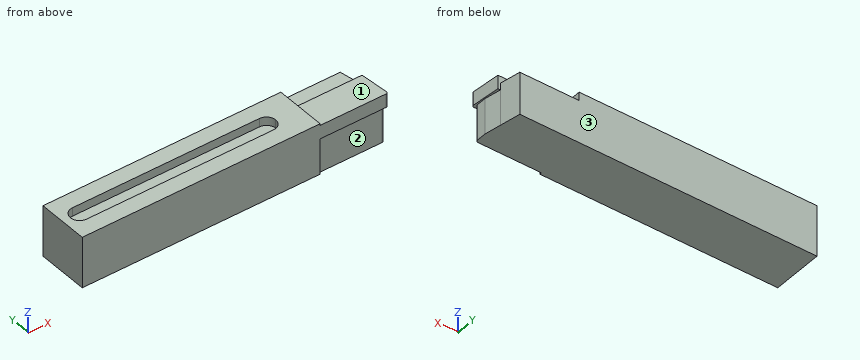
from build123d import *

# Parameters (mm, degrees)
F1_DEPTH = 9.525
F2_START = 6.35
F2_DEPTH = 6.35
F3_START = 3.81
F3_DEPTH = 5.08


with BuildPart() as f1:
    # F0 (on Top) → F1 (new body, symmetric)
    with BuildSketch(Plane.XY):
        Polygon((-57.15, 9.525), (-57.15, -9.525), (31.75, -9.525), (31.75, -8.73125), (31.75, 1.905), (31.75, 9.525), align=None)
        with BuildLine():
            ThreePointArc((-50.8, -3.429), (-54.229, 0), (-50.8, 3.429))
            Line((-50.8, 3.429), (19.05, 3.429))
            ThreePointArc((19.05, 3.429), (21.4746691527, 2.4246691527), (22.479, 0))
            ThreePointArc((22.479, 0), (21.4746691527, -2.4246691527), (19.05, -3.429))
            Line((19.05, -3.429), (-50.8, -3.429))
        make_face(mode=Mode.SUBTRACT)
        with BuildLine():
            Line((31.75, 1.905), (31.75, -8.73125))
            Line((31.75, -8.73125), (55.5625, -8.73125))
            ThreePointArc((55.5625, -8.73125), (56.1237660076, -8.4987660076), (56.35625, -7.9375))
            Line((56.35625, -7.9375), (56.35625, -4.2296700557))
            Line((56.35625, -4.2296700557), (55.2745421514, 1.905))
            Line((55.2745421514, 1.905), (31.75, 1.905))
        make_face()
        Polygon((53.9309305584, 9.525), (31.75, 9.525), (31.75, 1.905), (55.2745421514, 1.905), align=None)
        with BuildLine():
            ThreePointArc((-50.8, -3.429), (-48.3753308473, -2.4246691527), (-47.371, 0))
            ThreePointArc((-47.371, 0), (-48.3753308473, 2.4246691527), (-50.8, 3.429))
            ThreePointArc((-50.8, 3.429), (-54.229, 0), (-50.8, -3.429))
        make_face()
        with BuildLine():
            ThreePointArc((-50.8, 3.429), (-48.3753308473, 2.4246691527), (-47.371, 0))
            ThreePointArc((-47.371, 0), (-48.3753308473, -2.4246691527), (-50.8, -3.429))
            Line((-50.8, -3.429), (19.05, -3.429))
            ThreePointArc((19.05, -3.429), (15.621, 0), (19.05, 3.429))
            Line((19.05, 3.429), (-50.8, 3.429))
        make_face()
        with BuildLine():
            ThreePointArc((22.479, 0), (21.4746691527, 2.4246691527), (19.05, 3.429))
            ThreePointArc((19.05, 3.429), (15.621, 0), (19.05, -3.429))
            ThreePointArc((19.05, -3.429), (21.4746691527, -2.4246691527), (22.479, 0))
        make_face()
    extrude(amount=F1_DEPTH, both=True)

    # F0 (on Top) → F2 (cut)
    with BuildSketch(Plane.XY.offset(F2_START)):
        with BuildLine():
            Line((31.75, 1.905), (31.75, -8.73125))
            Line((31.75, -8.73125), (55.5625, -8.73125))
            ThreePointArc((55.5625, -8.73125), (56.1237660076, -8.4987660076), (56.35625, -7.9375))
            Line((56.35625, -7.9375), (56.35625, -4.2296700557))
            Line((56.35625, -4.2296700557), (55.2745421514, 1.905))
            Line((55.2745421514, 1.905), (31.75, 1.905))
        make_face()
        Polygon((53.9309305584, 9.525), (31.75, 9.525), (31.75, 1.905), (55.2745421514, 1.905), align=None)
        with BuildLine():
            ThreePointArc((-50.8, -3.429), (-48.3753308473, -2.4246691527), (-47.371, 0))
            ThreePointArc((-47.371, 0), (-48.3753308473, 2.4246691527), (-50.8, 3.429))
            ThreePointArc((-50.8, 3.429), (-54.229, 0), (-50.8, -3.429))
        make_face()
        with BuildLine():
            ThreePointArc((-50.8, 3.429), (-48.3753308473, 2.4246691527), (-47.371, 0))
            ThreePointArc((-47.371, 0), (-48.3753308473, -2.4246691527), (-50.8, -3.429))
            Line((-50.8, -3.429), (19.05, -3.429))
            ThreePointArc((19.05, -3.429), (15.621, 0), (19.05, 3.429))
            Line((19.05, 3.429), (-50.8, 3.429))
        make_face()
        with BuildLine():
            ThreePointArc((22.479, 0), (21.4746691527, 2.4246691527), (19.05, 3.429))
            ThreePointArc((19.05, 3.429), (15.621, 0), (19.05, -3.429))
            ThreePointArc((19.05, -3.429), (21.4746691527, -2.4246691527), (22.479, 0))
        make_face()
    extrude(amount=F2_DEPTH, mode=Mode.SUBTRACT)

    # F0 (on Top) → F3 (join)
    with BuildSketch(Plane.XY.offset(F3_START)):
        with BuildLine():
            Line((31.75, -8.73125), (31.75, -9.525))
            Line((31.75, -9.525), (56.35625, -9.525))
            ThreePointArc((56.35625, -9.525), (56.9175160076, -9.2925160076), (57.15, -8.73125))
            Line((57.15, -8.73125), (56.35625, -4.2296700557))
            Line((56.35625, -4.2296700557), (56.35625, -7.9375))
            ThreePointArc((56.35625, -7.9375), (56.1237660076, -8.4987660076), (55.5625, -8.73125))
            Line((55.5625, -8.73125), (31.75, -8.73125))
        make_face()
        with BuildLine():
            Line((31.75, 1.905), (31.75, -8.73125))
            Line((31.75, -8.73125), (55.5625, -8.73125))
            ThreePointArc((55.5625, -8.73125), (56.1237660076, -8.4987660076), (56.35625, -7.9375))
            Line((56.35625, -7.9375), (56.35625, -4.2296700557))
            Line((56.35625, -4.2296700557), (55.2745421514, 1.905))
            Line((55.2745421514, 1.905), (31.75, 1.905))
        make_face()
        Polygon((56.35625, -4.2296700557), (57.15, -8.73125), (56.2194487026, 1.905), (55.2745421514, 1.905), align=None)
    extrude(amount=F3_DEPTH)


solid = f1.part
Verification items for the finished model (mm, model axes). Face numbers are marked on the shaded views. A direction names the side the tool comes from. Give positions to 0.01 mm unless a question says otherwise; leave off trailing zeros. Loops run counter-clockwise (first coordinate to the right, second up) from the corner with the lowest first, then second, coordinate; pieces in that order, holes last. Notation, with made-up numbers: (-11.75, 13) - (-5.75, 13) arc R21 ccw to (-5.75, 35) - close; hole circle Ø6 at (65.25, 87). An arc over 180 degrees is marked (long way). Write item = value, one per line. Start each with the question number.
Q1. Tool access check on the marked faces 1, 2 and 3. Record the directions out of +Z, -Z, +X, -X, +Y, -Y that give a thin tool (end or side, any length) a straight path to the whole face; none if there is none.
Q2. Cross-section at C-C, the plane y = -1.75. Enter the section's corners in (x, z) (3 decimals), and give its area (3 significant figures).
Q3. Cross-section at D-D, the plane x = -8. Enter the section's corners in (y, z) (3 decimals), and give its area (3 significant figures).
Q4. Depth check by flat-ended pin: P1, Ø2, axis at y = -1, z = 4, coming from the +X side; P2, Ø3.5, axis at y = 3, z = 7.5, coming from the +X side; P3, Ø6, axis at y = -1.5, z = 4.5, coming from the +X side. Enter the tip coordinate at first touch or a pass-through.
Q5. Thickness scan on line 1 (Z direction, x = 36.5, y = -7) (3 decimals); line 2 (X direction, y = 1.5, z = 8.75); line 3 (X direction, y = 0.25, z = 5.5). Record the ranges inside material, lowest first.
Answer key:
q1.face_1 = +Z, +X, +Y, -Y
q1.face_2 = -Z, +X, -Y
q1.face_3 = +Z, -Z, +X, -X, +Y
q2.outline = (-57.15, -9.525) - (55.919, -9.525) - (55.919, 3.81) - (56.539, 3.81) - (56.539, 8.89) - (31.75, 8.89) - (31.75, 9.525) - (21.999, 9.525) - (21.999, 6.35) - (-53.749, 6.35) - (-53.749, 9.525) - (-57.15, 9.525) - close
q2.area = 1,900 mm^2
q3.outline = (-9.525, -9.525) - (9.525, -9.525) - (9.525, 9.525) - (3.429, 9.525) - (3.429, 6.35) - (-3.429, 6.35) - (-3.429, 9.525) - (-9.525, 9.525) - close
q3.area = 341 mm^2
q4.P1 = 56.56
q4.P2 = 56.28
q4.P3 = 56.78
q5.line_1 = -9.525 to 8.89
q5.line_2 = -57.15 to -53.88, 22.13 to 56.25
q5.line_3 = -57.15 to 56.36
